Autodesk Inventor part; units mm, degrees
ref_plane "YZ Plane" through (0, 0, 0) normal (1, 0, 0) x (0, 1, 0)
ref_plane "XZ Plane" through (0, 0, 0) normal (0, 1, 0) x (-1, 0, 0)
ref_plane "XY Plane" through (0, 0, 0) normal (0, 0, 1) x (1, 0, 0)
sketch "스케치1" plane through (0, 0, 0) normal (0, 0, 1) x (1, 0, 0)
  circle A0 centre (0, 0) radius 3
  arc A1 (-5, 0) -> (5, 0) centre (0, 0) ccw
  circle A2 centre (0, 17) radius 3
  line L0 (-5, 0) -> (8.6834, 0) construction
  line L1 (-40, 14) -> (-40, 20)
  line L2 (-40, 20) -> (-5.1962, 20)
  line L3 (5, 0) -> (5, 13.6834)
  line L4 (-40, 14) -> (-5, 14)
  line L5 (-5, 0) -> (-5, 14)
  arc A3 (5, 13.6834) -> (-5.1962, 20) centre (0, 17) ccw
  dimension "d2" = 6
  dimension "d4" = 17
  dimension "d5" = 10
  dimension "d7" = 6
  dimension "d9" = 6
  dimension "d10" = 40
  dimension "d12" = 14
  dimension "d13" = 6
extrude "돌출1" add sketch "스케치1" along normal mid plane 14
chamfer "모따기1" distance 1 angle 45 2 edges at (-40, 20, 0) (-40, 14, 0)
fillet "모깎기1" radius 8 3 edges at (-5, 14, 0) (-5.1962, 20, 0) (5, 13.6834, 0)
sketch "스케치2" plane through (-39, 20, 7) normal (0, 1, 0) x (1, 0, 0)
  circle A0 centre (10, 7) radius 3.5
  line L0 (0, 0) -> (0, 14)
  line L1 (30.3397, 0) -> (0, 0)
  point P0 (39, 7)
  dimension "d20" = 7
  dimension "d21" = 10
  dimension "d22" = 7
extrude "돌출2" cut sketch "스케치2" against normal blind 4
ref_plane "작업 평면1" through (0, 0, 0) normal (0, 0, 1) x (1, 0, 0)
sketch "스케치3" plane through (0, 0, 0) normal (0, 0, 1) x (1, 0, 0)
  line L0 (15.6771, 9) -> (-15.3905, 9)
  line L1 (-15.3905, 9) -> (-15.3905, -8.77)
  line L2 (-15.3905, -8.77) -> (15.6771, -8.77)
  line L3 (15.6771, -8.77) -> (15.6771, 9)
  arc A0 (-5, 0) -> (5, 0) centre (0, 0) ccw
  dimension "d25" = 14
extrude "돌출3" cut sketch "스케치3" along normal mid plane 6
sketch "스케치4" plane through (-39, 20, 7) normal (0, 1, 0) x (1, 0, 0)
  point P0 (39, 7)
properties part number "1번부품"
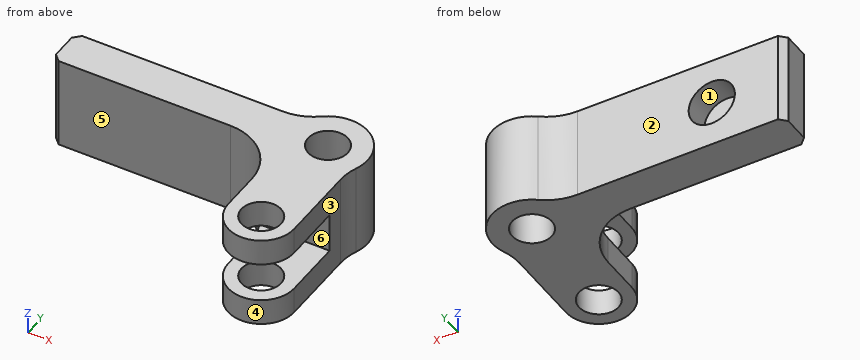
Geometry check sheet. Reference: the model listing, model coordinates, mm. Face numbers are marked on the shaded views. A direction names the side the tool comes from. Coordinates: 2 decimals unless noted, no trailing zeros. Order: outer loops, then holes, each group sorted by start corner. A loop starts at its lowest first (then second) coordinate and runs counter-clockwise, first axis right, second up. Notation, with made-up numbers: M 9,28.25 L 67,28.25 A15 cw 67,49.25 Z; hole C 5,34 d7. An arc over 180 degrees is marked long. Answer as a JSON object with one key per item and string values.
Q1. Cross-section at B-B on x = 0. Record the cut outline in (y, z), and give its area (3 significant figures).
Results are:
{"outline": "M -5,-7 L -3,-7 L -3,-3 L -5,-3 Z; M -5,3 L -3,3 L -3,7 L -5,7 Z; M 3,-7 L 14,-7 L 14,7 L 3,7 L 3,3 L 9,3 L 9,-3 L 3,-3 Z; M 20,-7 L 23,-7 L 23,7 L 20,7 Z", "area": "176 mm²"}
Q2. Tool access check on the marked faces 4, 5 and 6. Record the directions out of +Z, -Z, +X, -X, +Y, -Y that give a thin tool (end or side, any length) a straight path to the whole face; none if there is none.
Results are:
{"face 4": "+Z, -Z, -Y", "face 5": "+Z, -Z, -X, -Y", "face 6": "+X, -X, -Y"}
Q3. Cross-section at D-D on y = -2. Record the cut outline in (x, z).
Results are:
{"outline": "M -4.58,-7 L -2.24,-7 L -2.24,-3 L -4.58,-3 Z; M -4.58,3 L -2.24,3 L -2.24,7 L -4.58,7 Z; M 2.24,-7 L 4.58,-7 L 4.58,-3 L 2.24,-3 Z; M 2.24,3 L 4.58,3 L 4.58,7 L 2.24,7 Z"}
Q4. Depth check by flat-ended pin: pin 1 Ø4 at (x, z) = (-23, -1.5) entering from -Y; pin 2 Ø5 at (y, z) = (8.5, 4) entering from -X (3 decimals); pin 3 Ø1.5 at (y, z) = (15, -5) entering from +X. Enter the tip coordinate at first touch or a pass-through.
Results are:
{"pin 1": "stops at y = 14", "pin 2": "stops at x = -6.755", "pin 3": "stops at x = 5.87"}
Q5. Scan lines: line 1 (Y direction, x = 0, z = -4.7); line 2 (X direction, y = 0, z = -5.65); line 3 (X direction, y = 18.95, z = 0). Record each from-to range of solid material in increasing order.
Results are:
{"line 1": "y = -5 to -3, 3 to 14, 20 to 23", "line 2": "x = -5 to -3, 3 to 5", "line 3": "x = -40 to -32.5, -25.5 to -2.28, 2.28 to 5.67"}
Q6. Release check for a two-part mould opening along X. For the marked faces 1, 2 and 3 record: released by +X, released by -X, zero draft, split by the parting line, or undercut.
Results are:
{"face 1": "undercut", "face 2": "zero draft", "face 3": "released by +X"}
Q7. Cross-section at C-C on z = -4. Record the cut outline in (x, y).
Results are:
{"outline": "M -40,15 L -39,14 L -13,14 A8 cw -5,6 L -5,0 A5 ccw 5,0 L 5,11.8 A8 cw 5.57,14.77 A6 ccw -3.71,21.71 A8 cw -8.66,20 L -39,20 L -40,19 Z; hole C 0,0 d6; hole C 0,17 d6"}
Q8. Cross-section at A-A on y = 17. Record the cut outline in (x, z), and give its area (3 significant figures).
Results are:
{"outline": "M -40,-7 L -3,-7 L -3,7 L -40,7 Z; M 3,-7 L 6,-7 L 6,7 L 3,7 Z; hole C -29,0 d7", "area": "522 mm²"}
